Source: CAD feature listing. Evaluate the final solid. Frame: model axes, mm. Round coordinates to 2 decimals unless told otherwise and drop trailing zeros. Loops run counter-clockwise (first coordinate to the right, second up) from the corner with the lowest first, then second, coordinate; pieces in that order, holes last. Notation, with made-up numbers: M 65.25,39 L 95.25,39 A15 ccw 95.25,59 Z; hole C 63.5,-9 d9. An arc over 180 degrees is marked long. Write each question's results on one line, items separated by ' | '. Start each with the question number.
1. Section D-D on y = 0.6. Give the number of separate pieces and of enclosed holes in the cut face, and give its area (3 significant figures).
2. Contact query for a flat-ended pin moving along its axis: pin 1 Ø2.5 at (x, z) = (60, -15) entering from -Y. Output: stop coordinate, or through.
3. Ray query, line 1 (Z direction, x = 54, y = 1.1); line 2 (X direction, y = 0.75, z = 7); line 3 (X direction, y = 1.5, z = -15). Return the intervals inside material, ascending.
4. Draft query along X for faces 1 (the cylindrical face through (-61.464, 1.014, 14.239)), 2 (the flat face through (-1, 2, 0)), 3 (the cylindrical face through (52.885, 1.014, -8.216)). Return one class per face: released by +X, released by -X, zero draft, split by the parting line, or undercut.
5. Section A-A on z = -15. Output: boundary loops of the cut face in (x, y).
6. Section B-B on z = 7. Output: boundary loops of the cut face in (x, y), and give its area (3 significant figures).
7. Section C-C on x = -54. Output: boundary loops of the cut face in (y, z), and give its area (3 significant figures).
from build123d import *

# Parameters (mm, degrees)
SKETCH_1_W               = 150
SKETCH_1_H               = 45
EXTRUDE_1_DEPTH          = 2
CUT_EXTRUDE_1_REACH      = 80.328
SKETCH_2_R               = 1.65
MIRROR_2_COPY_1_REACH    = 80.328
MIRROR_2_COPY_1_SKETCH_R = 1.65


with BuildPart() as part:
    # Sketch 1 → Extrude 1 (new body)
    with BuildSketch(Plane(origin=(0, 0, 0), x_dir=(1, 0, 0), z_dir=(0, 1, 0))):
        Rectangle(SKETCH_1_W, SKETCH_1_H)
    extrude(amount=EXTRUDE_1_DEPTH)

    # Sketch 2 → Cut-Extrude 1 (cut, up to next)
    with BuildSketch(Plane(origin=(0, 2, 0), x_dir=(1, 0, 0), z_dir=(0, 1, 0)), mode=Mode.PRIVATE) as cut_extrude_1_sk1:
        with Locations(Location((-60, 15, 0), (0, 0, 270))):
            Circle(SKETCH_2_R)
    cut_extrude_1_tool1 = extrude(cut_extrude_1_sk1.sketch, amount=-CUT_EXTRUDE_1_REACH, mode=Mode.PRIVATE) & part.part
    # Sketch 2 → Cut-Extrude 1 (cut, up to next)
    with BuildSketch(Plane(origin=(0, 2, 0), x_dir=(1, 0, 0), z_dir=(0, 1, 0)), mode=Mode.PRIVATE) as cut_extrude_1_sk2:
        with Locations(Location((-66, 7, 0), (0, 0, 270))):
            Circle(SKETCH_2_R)
    cut_extrude_1_tool2 = extrude(cut_extrude_1_sk2.sketch, amount=-CUT_EXTRUDE_1_REACH, mode=Mode.PRIVATE) & part.part
    # Sketch 2 → Cut-Extrude 1 (cut, up to next)
    with BuildSketch(Plane(origin=(0, 2, 0), x_dir=(1, 0, 0), z_dir=(0, 1, 0)), mode=Mode.PRIVATE) as cut_extrude_1_sk3:
        with Locations(Location((-54, 7, 0), (0, 0, 270))):
            Circle(SKETCH_2_R)
    cut_extrude_1_tool3 = extrude(cut_extrude_1_sk3.sketch, amount=-CUT_EXTRUDE_1_REACH, mode=Mode.PRIVATE) & part.part
    cut_extrude_1_1 = cut_extrude_1_tool1.solids().sort_by_distance((-60, 2, -15))[0]
    add(cut_extrude_1_1, mode=Mode.SUBTRACT)
    cut_extrude_1_2 = cut_extrude_1_tool2.solids().sort_by_distance((-66, 2, -7))[0]
    add(cut_extrude_1_2, mode=Mode.SUBTRACT)
    cut_extrude_1_3 = cut_extrude_1_tool3.solids().sort_by_distance((-54, 2, -7))[0]
    add(cut_extrude_1_3, mode=Mode.SUBTRACT)
    cut_extrude_1 = cut_extrude_1_1 + cut_extrude_1_2 + cut_extrude_1_3  # Cut-Extrude 1 as one shape, for the pattern or mirror that repeats it

    # Mirror 1: Cut-Extrude 1 across plane
    add(cut_extrude_1.mirror(Plane.XY), mode=Mode.SUBTRACT)

    # Mirror 2: Cut-Extrude 1 across plane
    add(cut_extrude_1.mirror(Plane(origin=(0, 0, 0), x_dir=(0, 0, 1), z_dir=(1, 0, 0))), mode=Mode.SUBTRACT)

    # Mirror 2 copy 1 sketch → Mirror 2 copy 1 (cut, up to next)
    with BuildSketch(Plane(origin=(0, 2, 0), x_dir=(-1, 0, 0), z_dir=(0, 1, 0)), mode=Mode.PRIVATE) as mirror_2_copy_1_sk1:
        with Locations(Location((-60, 15, 0), (0, 0, 270))):
            Circle(MIRROR_2_COPY_1_SKETCH_R)
    mirror_2_copy_1_tool1 = extrude(mirror_2_copy_1_sk1.sketch, amount=-MIRROR_2_COPY_1_REACH, mode=Mode.PRIVATE) & part.part
    # Mirror 2 copy 1 sketch → Mirror 2 copy 1 (cut, up to next)
    with BuildSketch(Plane(origin=(0, 2, 0), x_dir=(-1, 0, 0), z_dir=(0, 1, 0)), mode=Mode.PRIVATE) as mirror_2_copy_1_sk2:
        with Locations(Location((-66, 7, 0), (0, 0, 270))):
            Circle(MIRROR_2_COPY_1_SKETCH_R)
    mirror_2_copy_1_tool2 = extrude(mirror_2_copy_1_sk2.sketch, amount=-MIRROR_2_COPY_1_REACH, mode=Mode.PRIVATE) & part.part
    # Mirror 2 copy 1 sketch → Mirror 2 copy 1 (cut, up to next)
    with BuildSketch(Plane(origin=(0, 2, 0), x_dir=(-1, 0, 0), z_dir=(0, 1, 0)), mode=Mode.PRIVATE) as mirror_2_copy_1_sk3:
        with Locations(Location((-54, 7, 0), (0, 0, 270))):
            Circle(MIRROR_2_COPY_1_SKETCH_R)
    mirror_2_copy_1_tool3 = extrude(mirror_2_copy_1_sk3.sketch, amount=-MIRROR_2_COPY_1_REACH, mode=Mode.PRIVATE) & part.part
    add(mirror_2_copy_1_tool1.solids().sort_by_distance((60, 2, 15))[0], mode=Mode.SUBTRACT)
    add(mirror_2_copy_1_tool2.solids().sort_by_distance((66, 2, 7))[0], mode=Mode.SUBTRACT)
    add(mirror_2_copy_1_tool3.solids().sort_by_distance((54, 2, 7))[0], mode=Mode.SUBTRACT)


solid = part.part
Taken from the geometry:
1) separate pieces: 1 | enclosed holes: 12 | area: 6,650 mm^2
2) pin 1: through
3) line 1: -22.5 to -8.65, -5.35 to 5.35, 8.65 to 22.5 | line 2: -75 to -67.65, -64.35 to -55.65, -52.35 to 52.35, 55.65 to 64.35, 67.65 to 75 | line 3: -75 to -61.65, -58.35 to 58.35, 61.65 to 75
4) face 1: undercut | face 2: zero draft | face 3: undercut
5) outline: M -75,0 L -61.65,0 L -61.65,2 L -75,2 Z; M -58.35,0 L 58.35,0 L 58.35,2 L -58.35,2 Z; M 61.65,0 L 75,0 L 75,2 L 61.65,2 Z
6) outline: M -75,0 L -67.65,0 L -67.65,2 L -75,2 Z; M -64.35,0 L -55.65,0 L -55.65,2 L -64.35,2 Z; M -52.35,0 L 52.35,0 L 52.35,2 L -52.35,2 Z; M 55.65,0 L 64.35,0 L 64.35,2 L 55.65,2 Z; M 67.65,0 L 75,0 L 75,2 L 67.65,2 Z | area: 274 mm^2
7) outline: M 0,-22.5 L 2,-22.5 L 2,-8.65 L 0,-8.65 Z; M 0,-5.35 L 2,-5.35 L 2,5.35 L 0,5.35 Z; M 0,8.65 L 2,8.65 L 2,22.5 L 0,22.5 Z | area: 76.8 mm^2
